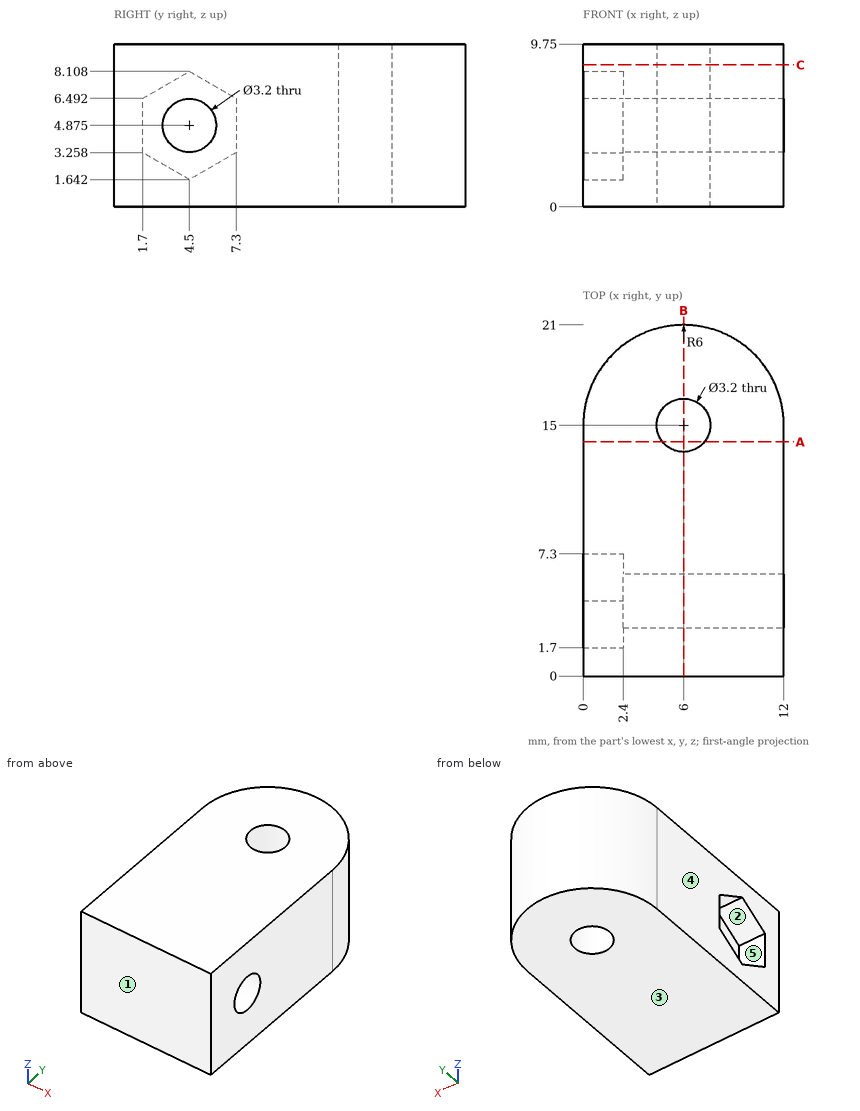
Part print with two shaded views. Sizes in mm from the minimum x, y, z corner. A direction names the side the tool comes from. Round coordinates to 2 decimals unless told otherwise and drop trailing zeros. Loops run counter-clockwise (first coordinate to the right, second up) from the corner with the lowest first, then second, coordinate; pieces in that order, holes last. Notation, with made-up numbers: M 21,66.5 L 27,66.5 A22 ccw 27,89.5 Z; hole C 15,74 d1. An arc over 180 degrees is marked long. Put each result on its own line as item: value. Start each with the question number.
Item 1: Drop flat-ended pins along their axis: P1, Ø3, axis at y = 4, z = 5.5, coming from the -X side; P2, Ø1.2, axis at x = 2, z = 5.5, coming from the +Y side. Give the stop position or say it passes through.
Item 2: Cut at C-C (z = 8.5). List the corners of the cut face in (x, y).
Item 3: Cut at A-A (y = 14). List the corners of the cut face in (x, z).
Item 4: Drill centre lines: line 1 along Y through (x, z) = (6, 6); line 2 along X through (y, z) = (15, 3); line 3 along Y through (x, z) = (4.75, 5) (1 decimal). Where is each one in solid material? Low to high.
Item 5: 3-axis set-ups, long thin cutter, end or side, ignore diameter. For the marked faces 1 and 2: which of +Z, -Z, +X, -X, +Y, -Y reach the whole face in a straight line?
Item 6: Mould opens along Z. For the marked faces 3, 4 and 5 say: released by +Z, released by -Z, zero draft, split by the parting line, or undercut.
Item 7: Cut at B-B (x = 6). Give the number of separate pieces and of enclosed holes in the cut face.
Answer block:
1. P1: x = 2.4
1. P2: y = 19.94
2. outline: M 0,0 L 12,0 L 12,15 A6 ccw 0,15 Z; hole C 6,15 d3.2
3. outline: M 0,0 L 4.75,0 L 4.75,9.75 L 0,9.75 Z; M 7.25,0 L 12,0 L 12,9.75 L 7.25,9.75 Z
4. line 1: 0 to 3.36, 5.64 to 13.4, 16.6 to 21
4. line 2: 0 to 4.4, 7.6 to 12
4. line 3: 0 to 2.9, 6.1 to 14, 16 to 20.9
5. face 1: +Z, -Z, +X, -X, -Y
5. face 2: -X
6. face 3: released by -Z
6. face 4: zero draft
6. face 5: undercut
7. separate pieces: 2
7. enclosed holes: 1
